The listing builds one solid part. Answer for the finished solid, in the listing's coordinates (mm). A direction names the side the tool comes from. Give positions to 0.01 mm unless a question says otherwise; leave off trailing zeros. Order: outer loops, then holes, each group sorted by start corner. A loop starts at its lowest first (then second) coordinate and runs counter-clockwise, first axis right, second up. Notation, with made-up numbers: (78, -30.75) - (99, -30.75) arc R10 ccw to (99, -16.75) - close; hole circle Ø7 at (46.25, 63.25). An arc over 180 degrees is marked (long way). Answer in a Markdown table with one row per item. Add a question column.
```python
from build123d import *

# Parameters (mm, degrees)
SKETCH_1_R          = 7.5
EXTRUDE_1_DEPTH     = 3
SKETCH_2_R          = 3.4
EXTRUDE_2_DEPTH     = 11.5
SKETCH_3_R          = 7.5
EXTRUDE_3_DEPTH     = 4
SKETCH_4_R          = 3.4
EXTRUDE_4_DEPTH     = 10
EXTRUDE_5_DEPTH     = 4
SKETCH_7_R          = 3.1
CUT_EXTRUDE_1_DEPTH = 11.5


with BuildPart() as part:
    # Эскиз1 → Бобышка-Вытянуть1 (new body)
    with BuildSketch(Plane.XY):
        Circle(SKETCH_1_R)
    extrude(amount=-EXTRUDE_1_DEPTH)

    # Эскиз2 → Бобышка-Вытянуть2 (add)
    with BuildSketch(Plane(origin=(0, 0, -3), x_dir=(-1, 0, 0), z_dir=(0, 0, -1))):
        Circle(SKETCH_2_R)
    extrude(amount=EXTRUDE_2_DEPTH)

    # Эскиз3 → Бобышка-Вытянуть3 (add)
    with BuildSketch(Plane(origin=(0, 0, -14.5), x_dir=(-1, 0, 0), z_dir=(0, 0, -1))):
        Circle(SKETCH_3_R)
    extrude(amount=-EXTRUDE_3_DEPTH)

    # Эскиз4 → Бобышка-Вытянуть4 (add)
    with BuildSketch(Plane(origin=(0, 0, -14.5), x_dir=(-1, 0, 0), z_dir=(0, 0, -1))):
        Circle(SKETCH_4_R)
    extrude(amount=EXTRUDE_4_DEPTH)

    # Эскиз6 → Бобышка-Вытянуть5 (add)
    with BuildSketch(Plane.XY.offset(-10.5)):
        with BuildLine():
            Line((-33.690694721, 51), (-33.690694721, 38))
            Line((-33.690694721, 38), (0, 4.775195955))
            Line((0, 4.775195955), (33.690694721, 38))
            Line((33.690694721, 38), (33.690694721, 51))
            Line((33.690694721, 51), (43.375005813, 51))
            Line((43.375005813, 51), (43.375005813, 38))
            Line((43.375005813, 38), (2.387366513, -2.420843062))
            ThreePointArc((2.387366513, -2.420843062), (0, -3.4), (-2.387366513, -2.420843062))
            Line((-2.387366513, -2.420843062), (-43.375005813, 38))
            Line((-43.375005813, 38), (-43.375005813, 51))
            Line((-43.375005813, 51), (-33.690694721, 51))
        make_face()
    extrude(amount=EXTRUDE_5_DEPTH)

    # Эскиз7 → Вырез-Вытянуть1 (cut, through all)
    with BuildSketch(Plane(origin=(0, 0, -10.5), x_dir=(-1, 0, 0), z_dir=(0, 0, -1))):
        with Locations((-38.532850267, 45)):
            Circle(SKETCH_7_R)
        with Locations((38.532850267, 45)):
            Circle(SKETCH_7_R)
    extrude(amount=-CUT_EXTRUDE_1_DEPTH, mode=Mode.SUBTRACT)


solid = part.part
```
(1) Find section A-A, the plane y = 45. Write down the section's boundary in (x, z) (3 decimals).
(2) For faces 1 (the face through (0, -4, -10.5)), 2 (the face through (0, 6, -10.5)), 3 (the face through (-1.6, -3, -5)), determine the directions among +Z, -Z, +X, -X, +Y, -Y from which every point of the face is accessible in a straight line to the end or side of a thin tool.
(3) Each of these flat-tipped pins is pushed along its axis until it touches: P1, Ø3, axis at x = 0.5, y = -2.5, coming from the +Z side; P2, Ø1.5, axis at x = 2.5, z = -4, coming from the +Y side; P3, Ø10, axis at x = 38.53, y = 45, coming from the +Z side; P4, Ø12, axis at y = 1.5, z = -20, coming from the +X side. Where does it stop, or does it pass through?
(4) Find section D-D, the plane y = 0. Write down the section's boundary in (x, z), plus the area to 3 significant figures.
(5) Find section C-C, the plane z = -4.75. Write down the section's boundary in (x, y).
(6) Find section B-B, the plane y = 29. Write down the section's boundary in (x, z), plus the area to 3 significant figures.
(7) Straight lines are drawn through the part: line 1 (Z direction, x = -26, y = 22); line 2 (X direction, y = 18.5, z = -7); line 3 (Y direction, x = 20, z = -7.75). For each, find the intervals that lie inside material, in ascending order.
(8) The mould has two halves that part along Z. Classify faces 4 (the face through (2, -3, -3)), 5 (the face through (-38.129, 48.074, -8.528)), 6 (the face through (0, 0, -24.5)): +Z half, -Z half, draft (parallel to the pull), parting line (faces both ways), or undercut.
Answer key:
| question | item | result |
|---|---|---|
| 1 | outline | (-43.375, -10.5) - (-41.633, -10.5) - (-41.633, -6.5) - (-43.375, -6.5) - close; (-35.433, -10.5) - (-33.691, -10.5) - (-33.691, -6.5) - (-35.433, -6.5) - close; (33.691, -10.5) - (35.433, -10.5) - (35.433, -6.5) - (33.691, -6.5) - close; (41.633, -10.5) - (43.375, -10.5) - (43.375, -6.5) - (41.633, -6.5) - close |
| 2 | face 1 | -Y |
| 2 | face 2 | +Y |
| 2 | face 3 | none |
| 3 | P1 | z = 0 |
| 3 | P2 | y = 2.92 |
| 3 | P3 | z = -6.5 |
| 3 | P4 | x = 7.5 |
| 4 | outline | (-7.5, -14.5) - (-3.4, -14.5) - (-3.4, -24.5) - (3.4, -24.5) - (3.4, -14.5) - (7.5, -14.5) - (7.5, -10.5) - (4.84, -10.5) - (4.84, -6.5) - (3.4, -6.5) - (3.4, -3) - (7.5, -3) - (7.5, 0) - (-7.5, 0) - (-7.5, -3) - (-3.4, -3) - (-3.4, -6.5) - (-4.84, -6.5) - (-4.84, -10.5) - (-7.5, -10.5) - close |
| 4 | area | 236 mm² |
| 5 | outline | circle Ø6.8 at (0, 0) |
| 6 | outline | (-34.25, -10.5) - (-24.56, -10.5) - (-24.56, -6.5) - (-34.25, -6.5) - close; (24.56, -10.5) - (34.25, -10.5) - (34.25, -6.5) - (24.56, -6.5) - close |
| 6 | area | 77.5 mm² |
| 7 | line 1 | -10.5 to -6.5 |
| 7 | line 2 | -23.6 to -13.92, 13.92 to 23.6 |
| 7 | line 3 | 14.95 to 24.5 |
| 8 | face 4 | undercut |
| 8 | face 5 | draft |
| 8 | face 6 | -Z half |
